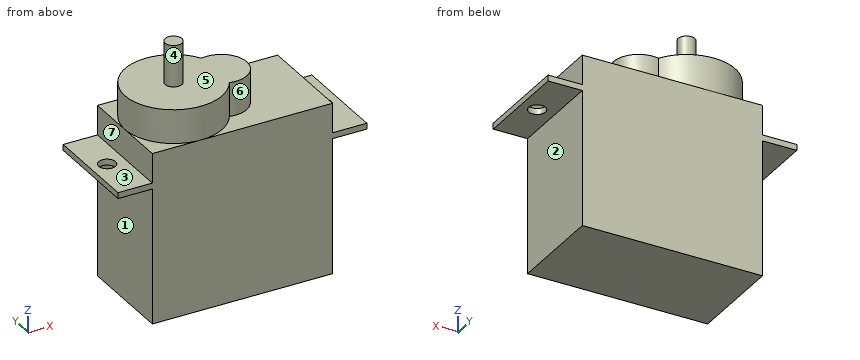
from build123d import *

# Parameters (mm, degrees)
F1_DEPTH = 11.5
F3_DEPTH = 4
F4_R     = 1
F5_DEPTH = 0.7
F6_R     = 1
F7_DEPTH = 0.7
F8_R     = 1
F9_DEPTH = 4.9


# Not quite as in the source:
# - a feature of the source that left no trace in its solid (it failed there, or was rolled back) is left out


with BuildPart() as f1:
    # F0 (on Front) → F1 (new body)
    with BuildSketch(Plane.XZ):
        Polygon((0, 16), (0, 0), (21.3, 0), (21.3, 16), (25.35, 16), (25.35, 16.7), (21.3, 16.7), (21.3, 20.2), (0, 20.2), (0, 16.7), (-4.05, 16.7), (-4.05, 16), align=None)
    extrude(amount=F1_DEPTH)

    # F2 (on face) → F3 (join)
    with BuildSketch(Plane.XY.offset(20.2)):
        with BuildLine():
            ThreePointArc((10.7044247788, -8.6682486377), (14.4, -5.75), (10.7044247788, -2.8317513623))
            ThreePointArc((10.7044247788, -2.8317513623), (0, -5.75), (10.7044247788, -8.6682486377))
        make_face()
    extrude(amount=F3_DEPTH)

    # F4 (on face) → F5 (cut, through all)
    with BuildSketch(Plane.XY.offset(16.7)):
        with Locations((-2.1, -5.75)):
            Circle(F4_R)
    extrude(amount=-F5_DEPTH, mode=Mode.SUBTRACT)

    # F6 (on face) → F7 (cut, through all)
    with BuildSketch(Plane.XY.offset(16.7)):
        with Locations((23.4, -5.75)):
            Circle(F6_R)
    extrude(amount=-F7_DEPTH, mode=Mode.SUBTRACT)

    # F8 (on face) → F9 (join)
    with BuildSketch(Plane.XY.offset(24.2)):
        with Locations((5.75, -5.75)):
            Circle(F8_R)
    extrude(amount=F9_DEPTH)


solid = f1.part
Verification items for the finished model (mm, model axes). Face numbers are marked on the shaded views. A direction names the side the tool comes from. Round coordinates to 2 decimals unless told otherwise and drop trailing zeros. Order: outer loops, then holes, each group sorted by start corner. A loop starts at its lowest first (then second) coordinate and runs counter-clockwise, first axis right, second up. Notation, with made-up numbers: (78.5, 51.5) -> (102.5, 51.5) arc R17 ccw to (102.5, 60.5) -> close; hole circle Ø3 at (31, 36). An arc over 180 degrees is marked (long way). Put each result on its own line as item: value.
1) Section check D-D (z = 15). Record the cut outline in (x, y), then the cut area to 3 significant figures.
Final values:
outline: (0, -11.5) -> (21.3, -11.5) -> (21.3, 0) -> (0, 0) -> close
area: 245 mm^2
2) Section check C-C (x = 11.4). Record the cut outline in (y, z), then the cut area to 3 significant figures.
Final values:
outline: (-11.5, 0) -> (0, 0) -> (0, 20.2) -> (-2.75, 20.2) -> (-2.75, 24.2) -> (-8.75, 24.2) -> (-8.75, 20.2) -> (-11.5, 20.2) -> close
area: 256 mm^2
3) Material ranges on line 1 (Y direction, x = 23.4, z = 16.55); line 2 (Z direction, x = -2.5, y = -4.5); line 3 (X direction, y = -1.5, z = 15.75), recorded low to high.
Final values:
line 1: y = -11.5 to -6.75, -4.75 to 0
line 2: z = 16 to 16.7
line 3: x = 0 to 21.3
4) Set-up check for the marked faces 1, 2, 3 and 4: record each of +Z, -Z, +X, -X, +Y, -Y from which the full face is reachable in a straight line by a thin tool's end or side.
Final values:
face 1: -Z, -X, +Y, -Y
face 2: -Z, +X, +Y, -Y
face 3: +Z, -X, +Y, -Y
face 4: +Z
5) Section check B-B (y = -5.25). Give the number of separate pieces and of enclosed holes in the cut face, then the cut area to 3 significant figures.
Final values:
separate pieces: 3
enclosed holes: 0
area: 499 mm^2
6) Section check A-A (x = 23.4). Record the cut outline in (y, z).
Final values:
outline: (-11.5, 16) -> (-6.75, 16) -> (-6.75, 16.7) -> (-11.5, 16.7) -> close; (-4.75, 16) -> (0, 16) -> (0, 16.7) -> (-4.75, 16.7) -> close
7) Depth check by flat-ended pin: pin 1 (1.5 mm diameter, centred on x = 12, z = 24, fed in from +Y); pin 2 (2.5 mm diameter, centred on x = -2.1, y = -5.75, fed in from +Z); pin 3 (4.5 mm diameter, centred on x = 22.5, y = -5.5, fed in from +Z); pin 4 (1.8 mm diameter, centred on x = 23.4, y = -5.75, fed in from -Z). Enter the tip coordinate at first touch or a pass-through.
Final values:
pin 1: stops at y = -2.75
pin 2: stops at z = 16.7
pin 3: stops at z = 20.2
pin 4: passes through
8) Mould release check, pull along X, two halves, no side actions. Record for the marked faces 5, 6 and 7: +X half, -X half, draft (parallel to the pull), parting line (faces both ways), or undercut.
Final values:
face 5: draft
face 6: undercut
face 7: -X half
